The model under review builds one solid part; all positions refer to its coordinate system, in mm. A direction names the side the tool comes from. Give positions to 0.01 mm unless a question says otherwise; leave off trailing zeros. Order: outer loops, then holes, each group sorted by start corner. A loop starts at its lowest first (then second) coordinate and runs counter-clockwise, first axis right, second up. Notation, with made-up numbers: (-4.5, -1) - (30.5, -1) arc R26 cw to (30.5, 21) - close; hole circle Ø3 at (81.25, 38). An arc over 180 degrees is marked (long way). Use a Markdown table: item, result. Add a question column.
```python
from build123d import *

# Parameters (mm, degrees)
BOSS_EXTRUDE1_DEPTH = 3.5
SKETCH2_W           = 20
SKETCH2_H           = 20
BOSS_EXTRUDE2_DEPTH = 3.5
SKETCH3_W           = 20
SKETCH3_H           = 3.5
BOSS_EXTRUDE3_DEPTH = 13.5
BOSS_EXTRUDE4_DEPTH = 3
SKETCH5_W           = 15.5
SKETCH5_H           = 6
BOSS_EXTRUDE5_DEPTH = 1.5
FILLET1_R           = 1
FILLET2_R           = 3
FILLET3_R           = 1.5
CUT_EXTRUDE1_DEPTH  = 3.5


with BuildPart() as part:
    # Sketch1 → Boss-Extrude1 (new body)
    with BuildSketch(Plane.XY):
        with BuildLine():
            Line((0, 0), (0, 15.5))
            ThreePointArc((0, 15.5), (0.292893219, 16.207106781), (1, 16.5))
            Line((1, 16.5), (32.6, 16.5))
            Line((32.6, 16.5), (32.6, 27.5))
            Line((32.6, 27.5), (-10.9, 27.5))
            Line((-10.9, 27.5), (-10.9, 0))
            Line((-10.9, 0), (0, 0))
        make_face()
    extrude(amount=BOSS_EXTRUDE1_DEPTH)

    # Sketch2 → Boss-Extrude2 (add)
    with BuildSketch(Plane.XZ):
        with Locations((-0.9, 10)):
            Rectangle(SKETCH2_W, SKETCH2_H)
    extrude(amount=BOSS_EXTRUDE2_DEPTH)

    # Sketch3 → Boss-Extrude3 (add)
    with BuildSketch(Plane.XZ.offset(3.5)):
        with Locations((-0.9, 18.25)):
            Rectangle(SKETCH3_W, SKETCH3_H)
    extrude(amount=BOSS_EXTRUDE3_DEPTH)

    # Sketch4 → Boss-Extrude4 (add)
    with BuildSketch(Plane(origin=(0, 27.5, 0), x_dir=(1, 0, 0), z_dir=(0, 1, 0))):
        Polygon((-10.9, 0), (-10.9, -3.5), (-10.9, -13), (4.6, -13), (4.6, -3.5), (4.6, 0), align=None)
    extrude(amount=BOSS_EXTRUDE4_DEPTH)

    # Sketch5 → Boss-Extrude5 (add)
    with BuildSketch(Plane.XY.offset(13)):
        with Locations((-3.15, 29)):
            Rectangle(SKETCH5_W, SKETCH5_H)
    extrude(amount=BOSS_EXTRUDE5_DEPTH)

    # Fillet1
    fillet1_edges = [part.edges().sort_by_distance(p)[0] for p in [
        (0, 0, 1.75),
    ]]
    fillet(fillet1_edges, radius=FILLET1_R)

    # Fillet2
    fillet2_edges = [part.edges().sort_by_distance(p)[0] for p in [
        (-4.95, 0, 3.5),
        (-3.15, 27.5, 3.5),
    ]]
    fillet(fillet2_edges, radius=FILLET2_R)

    # Fillet3
    fillet3_edges = [part.edges().sort_by_distance(p)[0] for p in [
        (9.1, -1.75, 0),
        (-0.9, -3.5, 16.5),
        (9.1, -17, 18.25),
        (-10.9, -17, 18.25),
        (4.6, 27.5, 1.75),
        (-3.15, 30.5, 0),
        (-0.9, 0, 20),
    ]]
    fillet(fillet3_edges, radius=FILLET3_R - 0.0001)  # a hair under: the kernel refuses the full size

    # Sketch6 → Cut-Extrude1 (cut)
    with BuildSketch(Plane(origin=(0, 0, 16.5), x_dir=(-1, 0, 0), z_dir=(0, 0, -1))):
        with BuildLine():
            ThreePointArc((5.1, -8.6), (3.261522369, -9.361522369), (2.5, -11.2))
            Line((2.5, -11.2), (7.7, -11.2))
            ThreePointArc((7.7, -11.2), (6.938477631, -9.361522369), (5.1, -8.6))
        make_face()
        with BuildLine():
            Line((7.7, -11.2), (2.5, -11.2))
            ThreePointArc((2.5, -11.2), (3.261522369, -13.038477631), (5.1, -13.8))
            ThreePointArc((5.1, -13.8), (6.938477631, -13.038477631), (7.7, -11.2))
        make_face()
        with BuildLine():
            ThreePointArc((5.1, -13.8), (3.261522369, -13.038477631), (2.5, -11.2))
            ThreePointArc((2.5, -11.2), (1.738477631, -13.038477631), (-0.1, -13.8))
            Line((-0.1, -13.8), (5.1, -13.8))
        make_face()
        with BuildLine():
            ThreePointArc((-0.1, -8.6), (1.738477631, -9.361522369), (2.5, -11.2))
            ThreePointArc((2.5, -11.2), (3.261522369, -9.361522369), (5.1, -8.6))
            Line((5.1, -8.6), (-0.1, -8.6))
        make_face()
        with BuildLine():
            ThreePointArc((-0.1, -13.8), (1.738477631, -13.038477631), (2.5, -11.2))
            Line((2.5, -11.2), (-2.7, -11.2))
            ThreePointArc((-2.7, -11.2), (-1.938477631, -13.038477631), (-0.1, -13.8))
        make_face()
        with BuildLine():
            Line((-2.7, -11.2), (2.5, -11.2))
            ThreePointArc((2.5, -11.2), (1.738477631, -9.361522369), (-0.1, -8.6))
            ThreePointArc((-0.1, -8.6), (-1.938477631, -9.361522369), (-2.7, -11.2))
        make_face()
    extrude(amount=-CUT_EXTRUDE1_DEPTH, mode=Mode.SUBTRACT)


solid = part.part
```
Q1. Wall thickness on probe 1 along Y at (x, z) = (5.5, 4.25); probe 2 along X at (y, z) = (8, 1.25); probe 3 along Z at (x, y) = (2, 23): over which ranges is each line inside the solid? List them lowest first.
Q2. We need section C-C (y = -12). Write out the cut boundary in (x, z), plus the area to 3 significant figures.
Q3. Draft analysis for pull direction Y (two halves, no side actions). For faces 6 (the cylindrical face through (-10.47, -16.55, 18.27)), 7 (the flat face through (-3, 29, 14.5)), 8 (the flat face through (-3, 27.5, 10)), state which applies: pulls with the +Y half, pulls with the -Y half, needs draft (parallel to the pull), parting line crosses it, or undercut.
Q4. Machinability: for faces 1 (the flat face through (4.6, 29, 9)), 2 (the flat face through (-3, 31, 13)), 3 (the flat face through (17, 16.5, 2)), 4 (the flat face through (-3, -8.6, 18)), 5 (the flat face through (6, 19, 3.5)), which of the approach directions +Z, -Z, +X, -X, +Y, -Y give a long, thin tool a straight path to every point of the face, cutting with its end or side? Answer none if there is none.
Q5. Clearance check with flat-ended pins moving along their axes: P1, Ø1.8, axis at x = 22, z = 2.5, coming from the +Y side; P2, Ø3, axis at x = -6.5, y = 30, coming from the +Z side; P3, Ø1, axis at x = -3.5, z = 18, coming from the +Y side. State where each tip first meets the part, or that it passes through.
Q6. We need section D-D (x = 2). Write out the cut boundary in (y, z), plus the area to 3 significant figures.
Q7. We need section A-A (x = -2.5). Write out the cut boundary in (y, z), plus the area to 3 significant figures.
Q8. We need section B-B (z = 10). Write out the cut boundary in (x, y).
Here are the results:
| question | item | result |
|---|---|---|
| 1 | probe 1 | -3.5 to 0 |
| 1 | probe 2 | -10.9 to 0 |
| 1 | probe 3 | 0 to 3.5 |
| 2 | outline | (-10.9, 16.5) - (-7.57, 16.5) - (-7.57, 20) - (-10.9, 20) - close; (2.57, 16.5) - (9.1, 16.5) - (9.1, 20) - (2.57, 20) - close |
| 2 | area | 34.5 mm2 |
| 3 | face 6 | pulls with the -Y half |
| 3 | face 7 | needs draft |
| 3 | face 8 | undercut |
| 4 | face 1 | +Z, +X, +Y |
| 4 | face 2 | -Z, +X, -X, +Y |
| 4 | face 3 | +Z, -Z, +X |
| 4 | face 4 | +Z, -Z |
| 4 | face 5 | +Z, +X |
| 5 | P1 | y = 27.5 |
| 5 | P2 | z = 14.5 |
| 5 | P3 | y = 0 |
| 6 | outline | (-17, 16.5) - (-12.97, 16.5) - (-12.97, 20) - (-17, 20) - close; (-9.43, 16.5) - (-5, 16.5) arc R1.5 cw to (-3.5, 15) - (-3.5, 0) - (0, 0) - (0, 18.5) arc R1.5 ccw to (-1.5, 20) - (-9.43, 20) - close; (16.5, 0) - (29, 0) arc R1.5 ccw to (30.5, 1.5) - (30.5, 13) - (32, 13) - (32, 14.5) - (26, 14.5) - (26, 13) - (27.5, 13) - (27.5, 6.5) arc R3 cw to (24.5, 3.5) - (16.5, 3.5) - close |
| 6 | area | 193 mm2 |
| 7 | outline | (-17, 16.5) - (-13.8, 16.5) - (-13.8, 20) - (-17, 20) - close; (-8.6, 16.5) - (-5, 16.5) arc R1.5 cw to (-3.5, 15) - (-3.5, 0) - (29, 0) arc R1.5 ccw to (30.5, 1.5) - (30.5, 13) - (32, 13) - (32, 14.5) - (26, 14.5) - (26, 13) - (27.5, 13) - (27.5, 6.5) arc R3 cw to (24.5, 3.5) - (3, 3.5) arc R3 cw to (0, 6.5) - (0, 18.5) arc R1.5 ccw to (-1.5, 20) - (-8.6, 20) - close |
| 7 | area | 247 mm2 |
| 8 | outline | (-10.9, -3.5) - (9.1, -3.5) - (9.1, 0) - (-10.9, 0) - close; (-10.9, 27.5) - (4.6, 27.5) - (4.6, 30.5) - (-10.9, 30.5) - close |
